from build123d import *

# Parameters (mm, degrees)
SKETCH1_R           = 1.5
BOSS_EXTRUDE1_DEPTH = 18
SKETCH2_W           = 1
SKETCH2_H           = 2
BOSS_EXTRUDE2_DEPTH = 2
CUT_EXTRUDE1_START  = -5
SKETCH3_W           = 2.236067978
SKETCH3_H           = 1
CUT_EXTRUDE1_DEPTH  = 2


with BuildPart() as part:
    # Sketch1 → Boss-Extrude1 (new body)
    with BuildSketch(Plane.XY):
        with Locations((-50, 6)):
            Circle(SKETCH1_R)
    extrude(amount=BOSS_EXTRUDE1_DEPTH)

    # Sketch2 → Boss-Extrude2 (add)
    with BuildSketch(Plane.XY.offset(18)):
        with Locations((-50, 6)):
            Rectangle(SKETCH2_W, SKETCH2_H)
    extrude(amount=BOSS_EXTRUDE2_DEPTH)

    # Sketch3 → Cut-Extrude1 (cut)
    with BuildSketch(Plane.XY.offset(18).offset(CUT_EXTRUDE1_START)):
        with Locations((-50, 7.5)):
            Rectangle(SKETCH3_W, SKETCH3_H)
    extrude(amount=-CUT_EXTRUDE1_DEPTH, mode=Mode.SUBTRACT)


solid = part.part
Read the model definition and answer for the solid it produces. Units are mm, in the model's axes. A direction names the side the tool comes from. Coordinates: 2 decimals unless noted, no trailing zeros. Order: outer loops, then holes, each group sorted by start corner. A loop starts at its lowest first (then second) coordinate and runs counter-clockwise, first axis right, second up. Notation, with made-up numbers: (76.5, -36) - (92.5, -36) arc R23 cw to (92.5, -6) - close; hole circle Ø10 at (-14, 62.25). An arc over 180 degrees is marked (long way). Use one line per item in the form item = value.
(1) Section B-B, the plane x = -50 is taken. Give the vertices of the cut face in (y, z), then the cut area to 3 significant figures.
Computed values:
outline = (4.5, 0) - (7.5, 0) - (7.5, 11) - (7, 11) - (7, 13) - (7.5, 13) - (7.5, 18) - (7, 18) - (7, 20) - (5, 20) - (5, 18) - (4.5, 18) - close
area = 57.0 mm²
(2) Section C-C, the plane z = 3.25 is taken. Give the vertices of the cut face in (x, y).
Computed values:
outline = circle Ø3 at (-50, 6)
(3) Which of the six approach directions +Z, -Z, +X, -X, +Y, -Y give full straight-line access (tool end or side, diameter ignored) to faces 1 (the face through (-49.5, 6, 19)), 2 (the face through (-50.5, 6, 19)), 3 (the face through (-50, 7, 19)), 4 (the face through (-50, 5, 19)), 5 (the face through (-50, 7, 12))?
Computed values:
face_1 = +Z, +X, +Y, -Y
face_2 = +Z, -X, +Y, -Y
face_3 = +Z, +X, -X, +Y
face_4 = +Z, +X, -X, -Y
face_5 = +X, -X, +Y
(4) Section A-A, the plane y = 6 is taken. Give the vertices of the cut face in (x, z), then the cut area to 3 significant figures.
Computed values:
outline = (-51.5, 0) - (-48.5, 0) - (-48.5, 18) - (-49.5, 18) - (-49.5, 20) - (-50.5, 20) - (-50.5, 18) - (-51.5, 18) - close
area = 56.0 mm²
(5) Straight lines are drawn through the part: L1, parallel to Z at x = -49.8, y = 4.85; L2, parallel to X at y = 6.1, z = 2.5; L3, parallel to Y at x = -50.4, z = 18.25. For each, find the intervals that lie inside material, in ascending order.
Computed values:
L1 = 0 to 18
L2 = -51.5 to -48.5
L3 = 5 to 7
(6) Given pin 1 Ø1.5 at (y, z) = (7, 4.5) entering from -X; pin 2 Ø0.6 at (x, z) = (-50, 12) entering from +Y; pin 3 Ø0.6 at (x, y) = (-50.5, 7.5) entering from +Z, each flat-ended and moving along its own axis, determine where each tip first touches the part or whether it passes through.
Computed values:
pin_1 = -51.48
pin_2 = 7
pin_3 = 18
(7) Section D-D, the plane y = 5.25 is taken. Give the vertices of the cut face in (x, z).
Computed values:
outline = (-51.3, 0) - (-48.7, 0) - (-48.7, 18) - (-49.5, 18) - (-49.5, 20) - (-50.5, 20) - (-50.5, 18) - (-51.3, 18) - close
